The listing builds one solid part. Answer for the finished solid, in the listing's coordinates (mm). A direction names the side the tool comes from. Coordinates: 2 decimals unless noted, no trailing zeros. Order: outer loops, then holes, each group sorted by start corner. A loop starts at its lowest first (then second) coordinate and runs counter-clockwise, first axis right, second up. Notation, with made-up numbers: (72, 56) -> (87, 56) arc R26 ccw to (87, 94) -> close; hole circle Ø6 at (22, -14.5). An arc over 180 degrees is marked (long way). Answer in a Markdown table with one row per item.
```python
from build123d import *

# Parameters (mm, degrees)
SKETCH_1_W          = 30
SKETCH_1_H          = 45
EXTRUDE_1_DEPTH     = 1.31
SKETCH_2_R          = 1.525
CUT_EXTRUDE_1_DEPTH = 10
SKETCH_3_W          = 14
SKETCH_3_H          = 37
CUT_EXTRUDE_2_DEPTH = 10
SKETCH_4_W          = 22
SKETCH_4_H          = 29
CUT_EXTRUDE_3_DEPTH = 10
FILLET_1_R          = 2
FILLET_2_R          = 2


with BuildPart() as part:
    # 草图1 → 凸台-拉伸1 (new body)
    with BuildSketch(Plane.XY):
        Rectangle(SKETCH_1_W, SKETCH_1_H)
    extrude(amount=EXTRUDE_1_DEPTH)

    # 草图2 → 切除-拉伸1 (cut)
    with BuildSketch(Plane.XY.offset(1.31)):
        with Locations((-10, 17.5)):
            Circle(SKETCH_2_R)
        with Locations((10, 17.5)):
            Circle(SKETCH_2_R)
        with Locations((-10, -17.5)):
            Circle(SKETCH_2_R)
        with Locations((10, -17.5)):
            Circle(SKETCH_2_R)
    extrude(amount=-CUT_EXTRUDE_1_DEPTH, mode=Mode.SUBTRACT)

    # 草图3 → 切除-拉伸2 (cut)
    with BuildSketch(Plane.XY.offset(1.31)):
        Rectangle(SKETCH_3_W, SKETCH_3_H)
    extrude(amount=-CUT_EXTRUDE_2_DEPTH, mode=Mode.SUBTRACT)

    # 草图4 → 切除-拉伸3 (cut)
    with BuildSketch(Plane.XY.offset(1.31)):
        Rectangle(SKETCH_4_W, SKETCH_4_H)
    extrude(amount=-CUT_EXTRUDE_3_DEPTH, mode=Mode.SUBTRACT)

    # 圆角1
    fillet_1_edges = [part.edges().sort_by_distance(p)[0] for p in [
        (-7, -18.5, 0.655),
        (11, -14.5, 0.655),
        (11, 14.5, 0.655),
        (7, 14.5, 0.655),
        (7, 18.5, 0.655),
        (-7, 18.5, 0.655),
        (-7, 14.5, 0.655),
        (-11, 14.5, 0.655),
        (-11, -14.5, 0.655),
        (-7, -14.5, 0.655),
        (7, -14.5, 0.655),
        (7, -18.5, 0.655),
    ]]
    fillet(fillet_1_edges, radius=FILLET_1_R - 0.0001)  # a hair under: the kernel refuses the full size

    # 圆角2
    fillet_2_edges = [part.edges().sort_by_distance(p)[0] for p in [
        (15, -22.5, 0.655),
        (-15, -22.5, 0.655),
        (-15, 22.5, 0.655),
        (15, 22.5, 0.655),
    ]]
    fillet(fillet_2_edges, radius=FILLET_2_R)


solid = part.part
```
(1) A cutting plane is placed at D-D, the plane x = 10.25. Determine the outline of the cut face in (y, z), then the cut area to 3 significant figures.
Check values:
| item | result |
|---|---|
| outline | (-22.5, 0) -> (-19, 0) -> (-19, 1.31) -> (-22.5, 1.31) -> close; (-16, 0) -> (-14.06, 0) -> (-14.06, 1.31) -> (-16, 1.31) -> close; (14.06, 0) -> (16, 0) -> (16, 1.31) -> (14.06, 1.31) -> close; (19, 0) -> (22.5, 0) -> (22.5, 1.31) -> (19, 1.31) -> close |
| area | 14.2 mm² |
(2) A cutting plane is placed at A-A, the plane y = 8. Determine the outline of the cut face in (x, z).
Check values:
| item | result |
|---|---|
| outline | (-15, 0) -> (-11, 0) -> (-11, 1.31) -> (-15, 1.31) -> close; (11, 0) -> (15, 0) -> (15, 1.31) -> (11, 1.31) -> close |
(3) Which of the six approach directions +Z, -Z, +X, -X, +Y, -Y give full straight-line access (tool end or side, diameter ignored) to faces 4 (the flat face through (0, -18.5, 1)), 5 (the flat face through (-14, 0, 0))?
Check values:
| item | result |
|---|---|
| face 4 | +Z, -Z |
| face 5 | -Z, +X, -X, +Y, -Y |
(4) A cutting plane is placed at B-B, the plane x = -0.75. Determine the outline of the cut face in (y, z).
Check values:
| item | result |
|---|---|
| outline | (-22.5, 0) -> (-18.5, 0) -> (-18.5, 1.31) -> (-22.5, 1.31) -> close; (18.5, 0) -> (22.5, 0) -> (22.5, 1.31) -> (18.5, 1.31) -> close |
(5) Find the intervals of material crossed by line 1 along Y through (x, z) = (4.25, 1.2); line 2 along Y through (x, z) = (10, 0.75) (3 decimals); line 3 along X through (y, z) = (-7.5, 0.7), in increasing order. Write a range as from..to.
Check values:
| item | result |
|---|---|
| line 1 | -22.5..-18.5, 18.5..22.5 |
| line 2 | -22.5..-19.025, -15.975..-14.232, 14.232..15.975, 19.025..22.5 |
| line 3 | -15..-11, 11..15 |
(6) For a pull along X with two mould halves and no side action, classify faces 1 (the flat face through (0, 22.5, 1)), 2 (the cylindrical face through (-14.43, 21.9, 0.66)), 3 (the flat face through (0, 18.5, 1)) as released by +X, released by -X, zero draft, split by the parting line, or undercut.
Check values:
| item | result |
|---|---|
| face 1 | zero draft |
| face 2 | released by -X |
| face 3 | undercut |
(7) A cutting plane is placed at C-C, the plane y = -17.5. Determine the outline of the cut face in (x, z) (3 decimals), then the cut area to 3 significant figures.
Check values:
| item | result |
|---|---|
| outline | (-15, 0) -> (-11.525, 0) -> (-11.525, 1.31) -> (-15, 1.31) -> close; (-8.475, 0) -> (-6.732, 0) -> (-6.732, 1.31) -> (-8.475, 1.31) -> close; (6.732, 0) -> (8.475, 0) -> (8.475, 1.31) -> (6.732, 1.31) -> close; (11.525, 0) -> (15, 0) -> (15, 1.31) -> (11.525, 1.31) -> close |
| area | 13.7 mm² |
